CAD build for the part. Positions are in the model's coordinates, mm. A direction names the side the tool comes from. Round coordinates to 2 decimals unless told otherwise and drop trailing zeros. Write each loop counter-clockwise with the first axis right and the second up, starting at its lowest first coordinate (ties: lowest second). Pieces come first, ordered by that corner, then holes. Notation, with made-up numbers: M 39,76.5 L 75,76.5 A35 ccw 75,114.5 Z; hole C 2.5,-6.75 d8. An arc over 180 degrees is marked long. Write each question's results on one line, items separated by ' | '. Start each with the question number.
```python
from build123d import *

# Parameters (mm, degrees)
F3_DEPTH = 1.5


with BuildPart() as f1:
    # F0 (on Front) → F1 (revolve)
    with BuildSketch(Plane.XZ):
        Polygon((0, 2.35), (0, 0), (15, 0), (15, 1.25), (1.5, 1.25), align=None)
    revolve(axis=Axis((7.5, 0, 0), (-1, 0, 0)))

    # F2 (on face) → F3 (cut)
    with BuildSketch(Plane(origin=(0, 0, 0), x_dir=(0, -1, 0), z_dir=(-1, 0, 0))):
        Polygon((0.57735, -1), (1.154701, 0), (0.57735, 1), (-0.57735, 1), (-1.154701, 0), (-0.57735, -1), align=None)
    extrude(amount=-F3_DEPTH, mode=Mode.SUBTRACT)


solid = f1.part
```
1) Saw through at A-A, the plane y = 0. Write the cut outline in (x, z), plus the area to 4 significant figures.
2) Saw through at B-B, the plane x = 10.75. Write the cut outline in (y, z), plus the area to 3 significant figures.
3) Drop flat-ended pins along their axis: pin 1 Ø1.5 at (x, y) = (5.5, 0) entering from -Z; pin 2 Ø1.3 at (x, y) = (1, 0) entering from -Z; pin 3 Ø0.6 at (x, y) = (0.5, -0.5) entering from +Z. Give the stop position or say it passes through.
4) 3-axis set-ups, long thin cutter, end or side, ignore diameter. For faces 4 (the face through (1, 0, 1)), 5 (the face through (15, 0, 0)): which of +Z, -Z, +X, -X, +Y, -Y reach the whole face in a straight line?
5) Pull direction Y, two halves, no side cores. Call faces 1 (the face through (8.16, -1.22, -0.27)), 2 (the face through (0.74, 0.86, 0.51)), 3 (the face through (0, -1, -1)): pulls with the +Y half, pulls with the -Y half, needs draft (parallel to the pull), parting line crosses it, or undercut.
6) Wall check: line 1 along X through (y, z) = (-0.15, 0.85); line 2 along Z through (x, y) = (9, 0.05); line 3 along Y through (x, z) = (6, 0.6). Give the ranges that are in metal, low to high. Write a range as from..to.
Filled sheet:
1) outline: M 0,-2.35 L 1.5,-1.25 L 15,-1.25 L 15,1.25 L 1.5,1.25 L 0,2.35 L 0,1 L 1.5,1 L 1.5,-1 L 0,-1 Z | area: 36.15 mm^2
2) outline: C 0,0 d2.5 | area: 4.91 mm^2
3) pin 1: stops at z = -1.25 | pin 2: stops at z = -2.09 | pin 3: stops at z = 2.15
4) face 4: -X | face 5: +Z, -Z, +X, +Y, -Y
5) face 1: parting line crosses it | face 2: undercut | face 3: needs draft
6) line 1: x = 1.5..15 | line 2: z = -1.25..1.25 | line 3: y = -1.1..1.1
